from build123d import *

# Parameters (mm, degrees)
SKETCH1_R           = 4
BOSS_EXTRUDE1_DEPTH = 5
SKETCH2_W           = 5
SKETCH2_H           = 35
BOSS_EXTRUDE2_DEPTH = 53.75
SKETCH3_W           = 75
SKETCH3_H           = 35
SKETCH3_R           = 2.55
BOSS_EXTRUDE3_DEPTH = 5
CHAMFER1_SIZE       = 45
CHAMFER1_SIZE2      = 32.69441376
FILLET1_R           = 4
FILLET2_START       = 98.583917136
FILLET2_DEPTH       = 28.75
FILLET2_START_2     = 25.643804114
FILLET2_2_DEPTH     = 87.749778627
SKETCH4_W           = 60
SKETCH4_H           = 5
CUT_EXTRUDE1_DEPTH  = 5


with BuildPart() as part:
    # Sketch1 → Boss-Extrude1 (new body)
    with BuildSketch(Plane(origin=(0, -83.529928381, 0), x_dir=(1, 0, 0), z_dir=(0, 1, 0))):
        with BuildLine():
            Line((103.583917136, -152.018693427), (122.333917136, -152.018693427))
            ThreePointArc((122.333917136, -152.018693427), (125.869451042, -150.554227333), (127.333917136, -147.018693427))
            Line((127.333917136, -147.018693427), (127.333917136, 7.981306573))
            ThreePointArc((127.333917136, 7.981306573), (125.869451042, 11.516840479), (122.333917136, 12.981306573))
            Line((122.333917136, 12.981306573), (103.583917136, 12.981306573))
            ThreePointArc((103.583917136, 12.981306573), (100.04838323, 11.516840479), (98.583917136, 7.981306573))
            Line((98.583917136, 7.981306573), (98.583917136, -147.018693427))
            ThreePointArc((98.583917136, -147.018693427), (100.04838323, -150.554227333), (103.583917136, -152.018693427))
        make_face()
        with Locations(Location((112.958917136, -142.018693427, 0), (0, 0, 180))):
            Circle(SKETCH1_R, mode=Mode.SUBTRACT)
        with Locations(Location((112.958917136, 2.981306573, 0), (0, 0, 180))):
            Circle(SKETCH1_R, mode=Mode.SUBTRACT)
    extrude(amount=BOSS_EXTRUDE1_DEPTH)

    # Sketch2 → Boss-Extrude2 (add)
    with BuildSketch(Plane(origin=(127.333917136, 0, 0), x_dir=(0, 0, -1), z_dir=(1, 0, 0))):
        with Locations((-109.518693427, -61.029928381)):
            Rectangle(SKETCH2_W, SKETCH2_H)
        with Locations((-29.518693427, -61.029928381)):
            Rectangle(SKETCH2_W, SKETCH2_H)
    extrude(amount=-BOSS_EXTRUDE2_DEPTH)

    # Sketch3 → Boss-Extrude3 (add)
    with BuildSketch(Plane.ZY.offset(-73.583917136)):
        with Locations((69.518693427, -61.029928381)):
            Rectangle(SKETCH3_W, SKETCH3_H)
        with Locations((49.718693427, -61.029928381)):
            Circle(SKETCH3_R, mode=Mode.SUBTRACT)
        with Locations((89.418693427, -61.029928381)):
            Circle(SKETCH3_R, mode=Mode.SUBTRACT)
        with Locations((89.418693427, -71.029928381)):
            Circle(SKETCH3_R, mode=Mode.SUBTRACT)
        with Locations((89.418693427, -51.029928381)):
            Circle(SKETCH3_R, mode=Mode.SUBTRACT)
        with Locations((49.718693427, -51.029928381)):
            Circle(SKETCH3_R, mode=Mode.SUBTRACT)
        with Locations((49.718693427, -71.029928381)):
            Circle(SKETCH3_R, mode=Mode.SUBTRACT)
        with Locations((59.568693427, -61.029928381)):
            Circle(SKETCH3_R, mode=Mode.SUBTRACT)
        with Locations((79.568693427, -61.029928381)):
            Circle(SKETCH3_R, mode=Mode.SUBTRACT)
    extrude(amount=-BOSS_EXTRUDE3_DEPTH)

    # Chamfer1
    chamfer1_edges = [part.edges().sort_by_distance(p)[0] for p in [
        (127.333917136, -43.529928381, 109.518693427),
        (127.333917136, -43.529928381, 29.518693427),
    ]]
    chamfer1_side = [part.faces().sort_by_distance(p)[0] for p in [
        (100.458917136, -43.529928381, 111.013006473),
    ]]
    chamfer(chamfer1_edges, length=CHAMFER1_SIZE, length2=CHAMFER1_SIZE2, reference=chamfer1_side[0])

    # Fillet1
    fillet1_edges = [part.edges().sort_by_distance(p)[0] for p in [
        (127.333917136, -76.224342141, 29.518693427),
        (127.333917136, -76.224342141, 109.518693427),
        (82.333917136, -43.529928381, 29.518693427),
        (82.333917136, -43.529928381, 109.518693427),
    ]]
    fillet(fillet1_edges, radius=FILLET1_R)

    # Fillet2: read off the stored shape, not the designer's step
    # Fillet2 outline → Fillet2 (add)
    with BuildSketch(Plane.YZ.offset(FILLET2_START)):
        with BuildLine():
            ThreePointArc((-78.529928381, 24.518693427), (-77.797695334, 26.28646038), (-76.029928381, 27.018693427))
            Line((-76.029928381, 27.018693427), (-78.529928381, 27.018693427))
            Line((-78.529928381, 27.018693427), (-78.529928381, 24.518693427))
        make_face()
        with BuildLine():
            ThreePointArc((-76.029928381, 32.018693427), (-77.797695334, 32.750926474), (-78.529928381, 34.518693427))
            Line((-78.529928381, 34.518693427), (-78.529928381, 32.018693427))
            Line((-78.529928381, 32.018693427), (-76.029928381, 32.018693427))
        make_face()
        with BuildLine():
            ThreePointArc((-78.529928381, 104.518693427), (-77.797695334, 106.28646038), (-76.029928381, 107.018693427))
            Line((-76.029928381, 107.018693427), (-78.529928381, 107.018693427))
            Line((-78.529928381, 107.018693427), (-78.529928381, 104.518693427))
        make_face()
        with BuildLine():
            ThreePointArc((-76.029928381, 112.018693427), (-77.797695334, 112.750926474), (-78.529928381, 114.518693427))
            Line((-78.529928381, 114.518693427), (-78.529928381, 112.018693427))
            Line((-78.529928381, 112.018693427), (-76.029928381, 112.018693427))
        make_face()
    extrude(amount=FILLET2_DEPTH)

    # Fillet2 2 outline → Fillet2 2 (cut)
    with BuildSketch(Plane.XY.offset(FILLET2_START_2)):
        with BuildLine():
            Line((127.333917136, -76.029928381), (126.652934202, -76.029928381))
            ThreePointArc((126.652934202, -76.029928381), (127.159885528, -77.095411005), (127.333917136, -78.262443939))
            Line((127.333917136, -78.262443939), (127.333917136, -76.029928381))
        make_face()
    extrude(amount=FILLET2_2_DEPTH, mode=Mode.SUBTRACT)

    # Sketch4 → Cut-Extrude1 (cut)
    with BuildSketch(Plane(origin=(78.583917136, 0, 0), x_dir=(0, 0, -1), z_dir=(1, 0, 0))):
        with Locations((-69.518693427, -43.529928381)):
            Rectangle(SKETCH4_W, SKETCH4_H)
        with Locations((-69.518693427, -78.529928381)):
            Rectangle(SKETCH4_W, SKETCH4_H)
    extrude(amount=-CUT_EXTRUDE1_DEPTH, mode=Mode.SUBTRACT)


solid = part.part
Model file for the job. Use its own axes, mm. A direction names the side the tool comes from. Round coordinates to 2 decimals unless told otherwise and drop trailing zeros. Order: outer loops, then holes, each group sorted by start corner. A loop starts at its lowest first (then second) coordinate and runs counter-clockwise, first axis right, second up. Notation, with made-up numbers: M 20.25,-29 L 29.25,-29 A9 cw 29.25,-24 Z; hole C 23,46 d6. An arc over 180 degrees is marked long. Write each question's results on one line, items separated by ' | '. Start each with the question number.
(1) Saw through at A-A, the plane z = 84.5. Give the cut face in (x, y).
(2) Saw through at C-C, the plane y = -80. Give the cut face in (x, z).
(3) Probe probe 1 along Z at (x, y) = (83.5, -58); probe 2 along X at (y, z) = (-55.5, 73); probe 3 along Y at (x, z) = (117.5, -6). List the from-to ranges inside material, lowest first. Write a range as from..to.
(4) Saw through at D-D, the plane x = 115. Give the cut face in (y, z).
(5) Saw through at B-B, the plane x = 91. Give the cut face in (y, z).
(6) Drop flat-ended pins along their axis: pin 1 (3 mm diameter, centred on y = -78.5, z = 84, fed in from -X); pin 2 (4 mm diameter, centred on x = 76.5, z = 79, fed in from -Y); pin 3 (23 mm diameter, centred on x = 118, z = -2, fed in from +Y); pin 4 (8 mm diameter, centred on x = 84.5, z = 64, fed in from -Y). Give the stop position or say it passes through.
(7) Two-plate mould, pull along Z, no slides. Class faces 1 (the face through (113, -81, 152.019)), 2 (the face through (113, -78.53, 6)), 3 (the face through (76.049, -59.307, 47.839)): pulls with the +Z half, pulls with the -Z half, needs draft (parallel to the pull), parting line crosses it, or undercut.
(8) Which spindle directions (+Z, -Z, +X, -X, +Y, -Y) get a long thin tool onto all of the face, cutting with end or side? Do faces 4 (the face through (76.049, -69.307, 47.839)), 5 (the face through (76, -43.53, 106)), 6 (the face through (83, -78.53, 30)), 7 (the face through (76, -76.03, 70)). Say none if no direction does.
Established:
1) outline: M 73.58,-76.03 L 78.58,-76.03 L 78.58,-46.03 L 73.58,-46.03 Z; M 98.58,-83.53 L 127.33,-83.53 L 127.33,-78.53 L 98.58,-78.53 Z
2) outline: M 98.58,-7.98 A5 ccw 103.58,-12.98 L 122.33,-12.98 A5 ccw 127.33,-7.98 L 127.33,147.02 A5 ccw 122.33,152.02 L 103.58,152.02 A5 ccw 98.58,147.02 Z; hole C 112.96,-2.98 d8; hole C 112.96,142.02 d8
3) probe 1: z = 27.02..32.02, 107.02..112.02 | probe 2: x = 73.58..78.58 | probe 3: y = -83.53..-78.53
4) outline: M -83.53,-12.98 L -78.53,-12.98 L -78.53,-6.42 L -83.53,-6.42 Z; M -83.53,0.46 L -78.53,0.46 L -78.53,24.52 A2.5 cw -76.03,27.02 L -67.26,27.02 L -67.26,32.02 L -76.03,32.02 A2.5 cw -78.53,34.52 L -78.53,104.52 A2.5 cw -76.03,107.02 L -67.26,107.02 L -67.26,112.02 L -76.03,112.02 A2.5 cw -78.53,114.52 L -78.53,138.58 L -83.53,138.58 Z; M -83.53,145.46 L -78.53,145.46 L -78.53,152.02 L -83.53,152.02 Z
5) outline: M -78.53,27.02 L -49.83,27.02 L -49.83,32.02 L -78.53,32.02 Z; M -78.53,107.02 L -49.83,107.02 L -49.83,112.02 L -78.53,112.02 Z
6) pin 1: stops at x = 98.58 | pin 2: stops at y = -76.03 | pin 3: stops at y = -78.53 | pin 4: passes through
7) face 1: pulls with the +Z half | face 2: needs draft | face 3: undercut
8) face 4: +X, -X | face 5: +Z, -Z, +X, -X, +Y | face 6: +Z, -Z, -X, -Y | face 7: +X, -X, -Y
